from build123d import *

# Parameters (mm, degrees)
SKETCH1_W               = 13.064472239
SKETCH1_H               = 20.176787348
BOSS_EXTRUDE1_DEPTH     = 5
SKETCH2_W               = 51
SKETCH2_H               = 73.5
BOSS_EXTRUDE2_DEPTH     = 2
SKETCH3_W               = 30
SKETCH3_H               = 25
BOSS_EXTRUDE3_DEPTH     = 10.5
SKETCH7_R               = 3.125
BOSS_EXTRUDE5_DEPTH     = 6.5
SKETCH8_W               = 4.189265903
SKETCH8_H               = 8
BOSS_EXTRUDE6_DEPTH     = 4
CUT_EXTRUDE1_DEPTH      = 70.538782979
CUT_EXTRUDE1_DEPTH_BACK = 70.538782979
SKETCH9_R               = 1.75


with BuildPart() as part:
    # Sketch1 → Boss-Extrude1 (new body)
    with BuildSketch(Plane(origin=(0, 0, 0), x_dir=(1, 0, 0), z_dir=(0, 1, 0))):
        with Locations((-6.53223612, 10.088393674)):
            Rectangle(SKETCH1_W, SKETCH1_H)
    extrude(amount=BOSS_EXTRUDE1_DEPTH)

    # Sketch2 → Boss-Extrude2 (add)
    with BuildSketch(Plane(origin=(0, 5, 0), x_dir=(1, 0, 0), z_dir=(0, 1, 0))):
        with Locations((-6.53223612, 20.176787348)):
            Rectangle(SKETCH2_W, SKETCH2_H)
    extrude(amount=BOSS_EXTRUDE2_DEPTH)

    # Sketch3 → Boss-Extrude3 (add)
    with BuildSketch(Plane(origin=(0, 7, 0), x_dir=(1, 0, 0), z_dir=(0, 1, 0))):
        with Locations((-17.03223612, 42.926787348)):
            Rectangle(SKETCH3_W, SKETCH3_H)
    extrude(amount=BOSS_EXTRUDE3_DEPTH)

    # Sketch7 → Boss-Extrude5 (add)
    with BuildSketch(Plane.ZY.offset(32.03223612)):
        with Locations(Location((-42.926787348, 14.375, 0), (0, 0, 90))):
            Circle(SKETCH7_R)
    extrude(amount=BOSS_EXTRUDE5_DEPTH)

    # Sketch8 → Boss-Extrude6 (add)
    with BuildSketch(Plane(origin=(0, 7, 0), x_dir=(1, 0, 0), z_dir=(0, 1, 0))):
        with Locations((16.873130929, 49.926787348)):
            Rectangle(SKETCH8_W, SKETCH8_H)
    extrude(amount=BOSS_EXTRUDE6_DEPTH)

    # Sketch9 → Cut-Extrude1 (cut, two sides: drawn at the far end of the back side and taken through both)
    with BuildSketch(Plane(origin=(0, 7, 0), x_dir=(1, 0, 0), z_dir=(0, 1, 0)).offset(-CUT_EXTRUDE1_DEPTH_BACK)):
        with Locations(Location((11.71776388, -14.063212652, 0), (0, 0, 270))):
            Circle(SKETCH9_R)
        with Locations(Location((-29.03223612, 53.926787348, 0), (0, 0, 270))):
            Circle(SKETCH9_R)
    extrude(amount=CUT_EXTRUDE1_DEPTH + CUT_EXTRUDE1_DEPTH_BACK, mode=Mode.SUBTRACT)


solid = part.part
Work out the finished part from the listing and answer in its coordinate system (mm). A direction names the side the tool comes from. Round coordinates to 2 decimals unless told otherwise and drop trailing zeros. Loops run counter-clockwise (first coordinate to the right, second up) from the corner with the lowest first, then second, coordinate; pieces in that order, holes last. Notation, with made-up numbers: M 85.25,25.5 L 91.25,25.5 A19 cw 91.25,39.5 Z; hole C -33.75,51.25 d8. An arc over 180 degrees is marked long. One line per question, with ' | ' between items. Start each with the question number.
(1) Find the intervals of material crossed by line 1 (Y direction, x = 8.5, z = -44.5); line 2 (Y direction, x = -9, z = -0.5); line 3 (X direction, y = 5.25, z = 4.5), in increasing order.
(2) For a pull along X with two mould halves and no side action, classify faces 5 (the face through (-29.7, 11.16, -52.31)), 6 (the face through (-32.032, 10, -36)), 7 (the face through (-7, 2, 0)) as released by +X, released by -X, zero draft, split by the parting line, or undercut.
(3) A cutting plane is placed at D-D on y = 13.5. Write down the section's boundary in (x, z), plus the area to 3 significant figures.
(4) A cutting plane is placed at B-B on x = -24.5. Write down the section's boundary in (y, z).
(5) A cutting plane is placed at A-A on y = 9.5. Write down the section's boundary in (x, z).
(6) Flat-ended cylindrical pins translate along their axes: pin 1 Ø5.5 at (x, y) = (-4, 2) entering from -Z; pin 2 Ø1 at (x, y) = (-31.5, 10.5) entering from -Z; pin 3 Ø2 at (y, z) = (8, -49.5) entering from -X; pin 4 Ø4 at (y, z) = (14.5, -26.5) entering from -X. Find the tip coordinate at first contact, or state that the pin passes through.
(7) A cutting plane is placed at C-C on z = -17. Write down the section's boundary in (x, y), plus the area to 3 significant figures.
(8) A tool of negligible diameter and unlimited length cuts with its end or side. For faces 1 (the face through (-35.237, 13.698, -39.876)), 2 (the face through (17, 9, -53.927)), 3 (the face through (17, 11, -50)), 4 (the face through (14.778, 9, -50)), from which of +Z, -Z, +X, -X, +Y, -Y can it reach the whole face along a straight path? Write none if from no direction.
Geometry check:
1) line 1: y = 5 to 7 | line 2: y = 0 to 7 | line 3: x = -32.03 to 18.97
2) face 5: undercut | face 6: released by -X | face 7: zero draft
3) outline: M -38.53,-45.93 L -32.03,-45.93 L -32.03,-55.43 L -29.93,-55.43 A1.75 cw long -28.13,-55.43 L -2.03,-55.43 L -2.03,-30.43 L -32.03,-30.43 L -32.03,-39.93 L -38.53,-39.93 Z | area: 780 mm²
4) outline: M 5,-56.93 L 7,-56.93 L 7,-55.43 L 17.5,-55.43 L 17.5,-30.43 L 7,-30.43 L 7,16.57 L 5,16.57 Z
5) outline: M -32.03,-55.43 L -29.93,-55.43 A1.75 cw long -28.13,-55.43 L -2.03,-55.43 L -2.03,-30.43 L -32.03,-30.43 Z; M 14.78,-53.93 L 18.97,-53.93 L 18.97,-45.93 L 14.78,-45.93 Z
6) pin 1: stops at z = -20.18 | pin 2: stops at z = -55.43 | pin 3: stops at x = -32.03 | pin 4: passes through
7) outline: M -32.03,5 L -13.06,5 L -13.06,0 L 0,0 L 0,5 L 18.97,5 L 18.97,7 L -32.03,7 Z | area: 167 mm²
8) face 1: -X | face 2: -Z, +X, +Y | face 3: +Z, -Z, +X, +Y | face 4: +Z, -Z, +Y
